Part print with two shaded views. Sizes in mm from the minimum x, y, z corner. A direction names the side the tool comes from. Give positions to 0.01 mm unless a question says otherwise; leave off trailing zeros. Write each loop counter-clockwise with the first axis right and the second up, starting at its lowest first coordinate (ties: lowest second). Pieces come first, ordered by that corner, then holes. Notation, with made-up numbers: (3, 11.25) - (41, 11.25) arc R8 ccw to (41, 25.25) - close; hole circle Ø2 at (-34, -19.75). An arc over 180 degrees is marked (long way). One line per item, written item: value. Start each with the question number.
(1) Drop flat-ended pins along their axis: P1, Ø12, axis at x = 30, y = 11, coming from the -Z side; P2, Ø12, axis at x = 36, z = 62.5, coming from the -Y side; P3, Ø3, axis at x = 21, y = 17, coming from the +Z side; P4, Ø2, axis at x = 7.5, y = 14, coming from the +Z side (3 decimals). Give the stop position or say it passes through.
(2) Cut at A-A, the plane z = 95. List the corners of the cut face in (x, y).
(3) Cut at C-C, the plane x = 29. List the corners of the cut face in (y, z), and give its area (3 significant figures).
(4) Cut at B-B, the plane y = 14. List the corners of the cut face in (x, z), and give its area (3 significant figures).
(5) 3-axis set-ups, long thin cutter, end or side, ignore diameter. For the marked faces 1 and 2: which of +Z, -Z, +X, -X, +Y, -Y reach the whole face in a straight line?
(6) Cut at D-D, the plane z = 61. List the corners of the cut face in (x, y), and give its area (3 significant figures).
(7) Mould opens along X. For the marked faces 3, 4, 5 and 6 say: pulls with the +X half, pulls with the -X half, needs draft (parallel to the pull), parting line crosses it, or undercut.
(8) Probe L1, parallel to X at y = 19, z = 47.5; L2, parallel to X at y = 14.75, z = 18; L3, parallel to Y at x = 10, z = 83.5. List the from-to ranges inside material, lowest first.
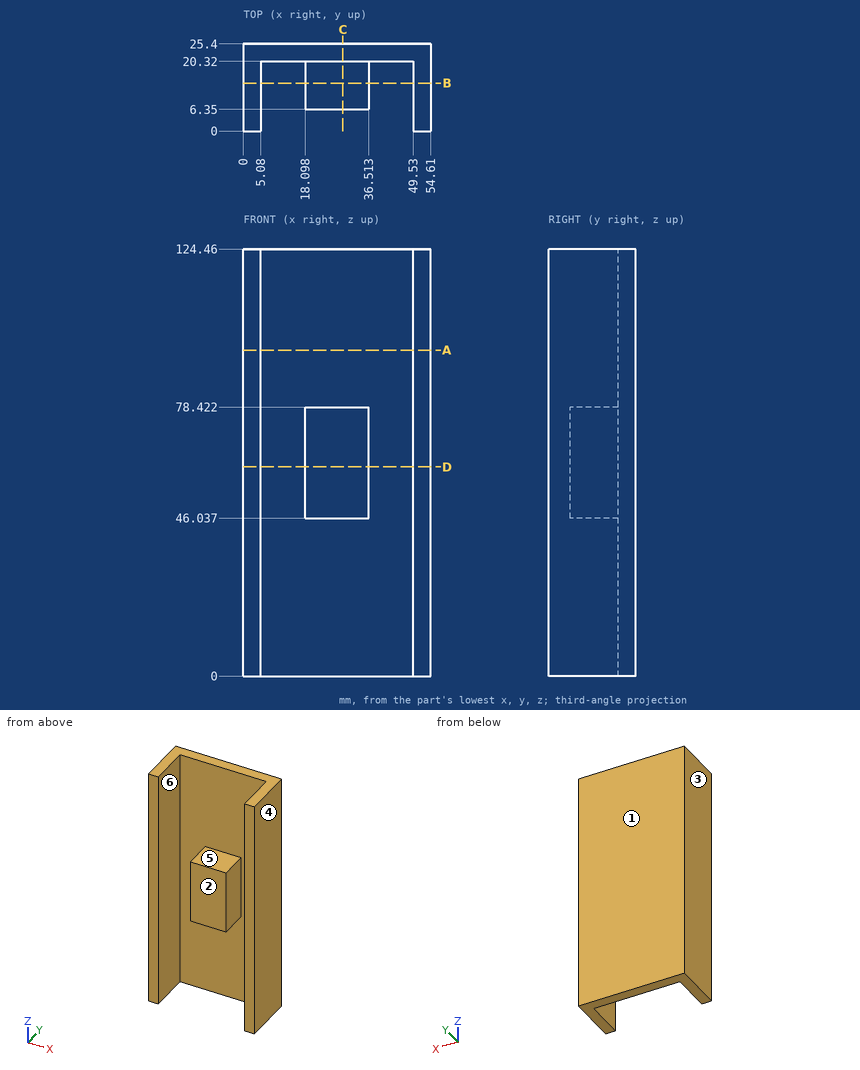
Answers follow:
1. P1: stops at z = 46.04
1. P2: stops at y = 6.35
1. P3: stops at z = 78.42
1. P4: passes through
2. outline: (0, 0) - (5.08, 0) - (5.08, 20.32) - (49.53, 20.32) - (49.53, 0) - (54.61, 0) - (54.61, 25.4) - (0, 25.4) - close
3. outline: (6.35, 46.04) - (20.32, 46.04) - (20.32, 0) - (25.4, 0) - (25.4, 124.46) - (20.32, 124.46) - (20.32, 78.42) - (6.35, 78.42) - close
3. area: 1,080 mm²
4. outline: (0, 0) - (5.08, 0) - (5.08, 124.46) - (0, 124.46) - close; (18.1, 46.04) - (36.51, 46.04) - (36.51, 78.42) - (18.1, 78.42) - close; (49.53, 0) - (54.61, 0) - (54.61, 124.46) - (49.53, 124.46) - close
4. area: 1,860 mm²
5. face 1: +Z, -Z, +X, -X, +Y
5. face 2: +Z, -Z, -Y
6. outline: (0, 0) - (5.08, 0) - (5.08, 20.32) - (18.1, 20.32) - (18.1, 6.35) - (36.51, 6.35) - (36.51, 20.32) - (49.53, 20.32) - (49.53, 0) - (54.61, 0) - (54.61, 25.4) - (0, 25.4) - close
6. area: 741 mm²
7. face 3: pulls with the -X half
7. face 4: pulls with the +X half
7. face 5: undercut
7. face 6: undercut
8. L1: x = 0 to 5.08, 18.1 to 36.51, 49.53 to 54.61
8. L2: x = 0 to 5.08, 49.53 to 54.61
8. L3: y = 20.32 to 25.4
